Verification items for this drawing (mm, ordinates from the low corner). A direction names the side the tool comes from. Coordinates: 2 decimals unless noted, no trailing zeros. Order: outer loops, then holes, each group sorted by start corner. A loop starts at its lowest first (then second) coordinate and runs counter-clockwise, first axis right, second up. Notation, with made-up numbers: M -19,-35 L 2,-35 A10 ccw 2,-17 Z; hole C -4,17 d5. An arc over 180 degrees is marked long. Write item = value, one per line.
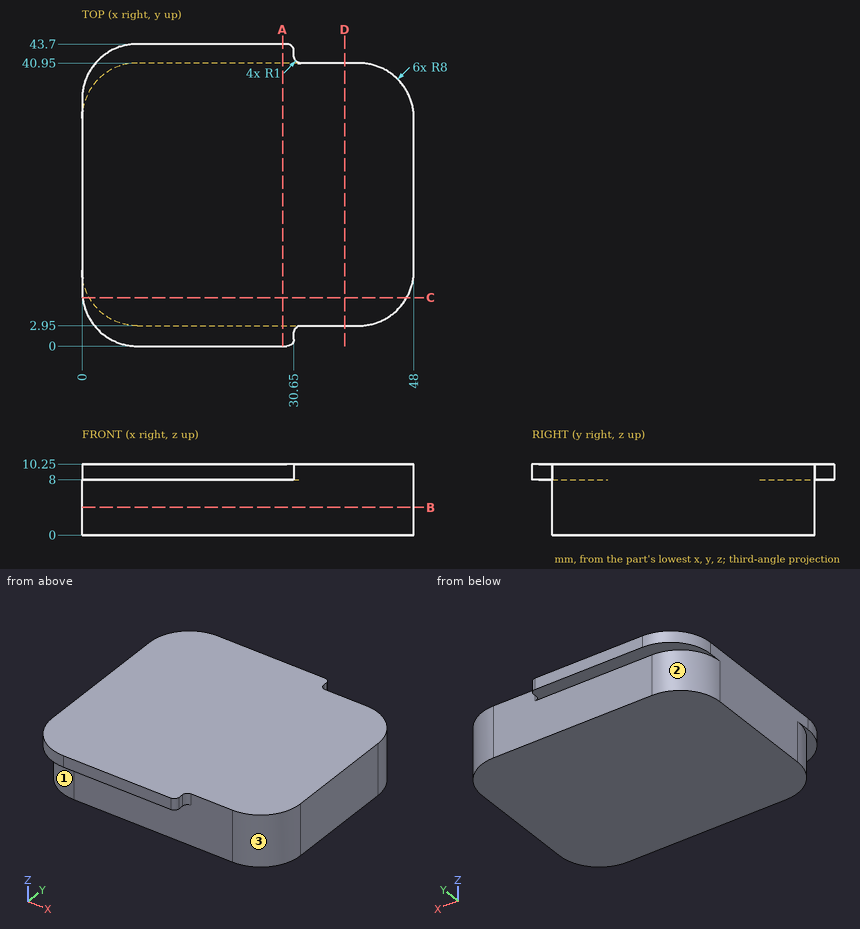
Item 1: Scan lines: L1, parallel to Y at x = 34, z = 1.75; L2, parallel to Y at x = 5.5, z = 0.5; L3, parallel to X at y = 34, z = 7.5. Record each from-to range of solid material in increasing order. Write a range as from..to.
Report:
L1 = 2.95..40.95
L2 = 3.35..40.55
L3 = 0.07..47.93
Item 2: Sectioned sample at C-C, the plane y = 7. Enter the section's corners in (x, z), then the cut area to 3 significant figures.
Report:
outline = M 0.06,8 L 1.04,8 L 1.04,0 L 46.96,0 L 46.96,10.25 L 0.06,10.25 Z
area = 473 mm^2
Item 3: Tool access check on the marked faces 1, 2 and 3. Record the directions out of +Z, -Z, +X, -X, +Y, -Y that give a thin tool (end or side, any length) a straight path to the whole face; none if there is none.
Report:
face_1 = -Z, -X, -Y
face_2 = -Z, -X, +Y
face_3 = +Z, -Z, +X, -Y
Item 4: Sectioned sample at B-B, the plane z = 4. Enter the section's corners in (x, y), then the cut area to 3 significant figures.
Report:
outline = M 0,10.95 A8 ccw 8,2.95 L 40,2.95 A8 ccw 48,10.95 L 48,32.95 A8 ccw 40,40.95 L 8,40.95 A8 ccw 0,32.95 Z
area = 1,770 mm^2
Item 5: Gauge pin test, flat ends, axial feed: pin 1 (1.5 mm diameter, centred on x = 37.5, z = 4.5, fed in from -Y); pin 2 (0.5 mm diameter, centred on y = 1.5, z = 9.5, fed in from +X); pin 3 (3.5 mm diameter, centred on x = 14, y = 5.5, fed in from -Z); pin 4 (3 mm diameter, centred on x = 12.5, z = 1.5, fed in from +Y). Record the tip position at first contact, or that the pin passes through.
Report:
pin_1 = 2.95
pin_2 = 30.65
pin_3 = 0
pin_4 = 40.95
Item 6: Sectioned sample at D-D, the plane x = 38. Enter the section's corners in (y, z).
Report:
outline = M 2.95,0 L 40.95,0 L 40.95,10.25 L 2.95,10.25 Z
Item 7: Sectioned sample at A-A, the plane x = 29. Enter the section's corners in (y, z).
Report:
outline = M 0,8 L 2.95,8 L 2.95,0 L 40.95,0 L 40.95,8 L 43.7,8 L 43.7,10.25 L 0,10.25 Z
